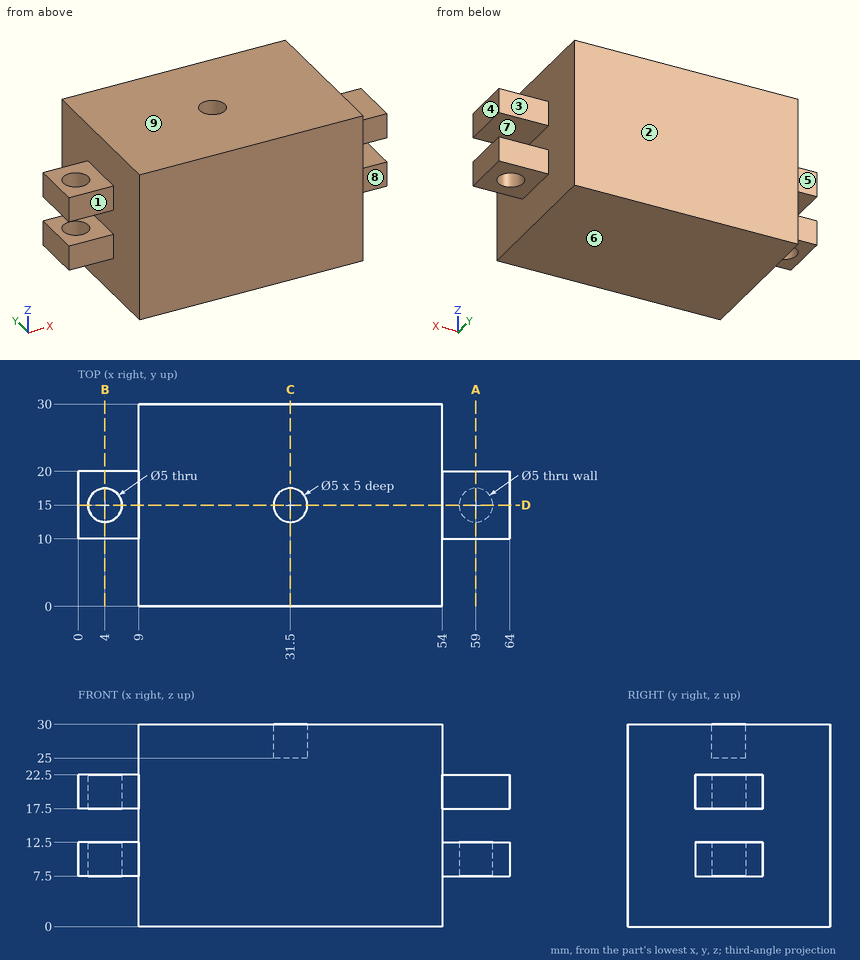
Print and shaded views of the part. All mm, measured from the part's lowest x, y and z. A direction names the side the tool comes from. Give positions to 0.01 mm unless a question says otherwise; leave off trailing zeros. Order: outer loops, then holes, each group sorted by start corner. A loop starts at its lowest first (then second) coordinate and runs counter-clockwise, first axis right, second up. Notation, with made-up numbers: (-28, 5) - (16, 5) arc R12 cw to (16, 28) - close; hole circle Ø4 at (78, 38.25). An arc over 180 degrees is marked (long way). Use a Markdown table: item, result.
1) 3-axis set-ups, long thin cutter, end or side, ignore diameter. For the marked faces 1, 2, 3, 4 and 5: which of +Z, -Z, +X, -X, +Y, -Y reach the whole face in a straight line?
Checked values:
| item | result |
|---|---|
| face 1 | +Z, -Z, -X, -Y |
| face 2 | +Z, -Z, +X, -X, +Y |
| face 3 | +Z, -Z, +X, +Y |
| face 4 | +Z, -Z, +X, +Y, -Y |
| face 5 | +Z, -Z, -X, +Y |
2) Flat gauge pins, fed straight in: P1, Ø4.5, axis at x = 4, y = 15, coming from the -Z side; P2, Ø2, axis at y = 25.5, z = 24.5, coming from the -X side; P3, Ø2.5, axis at x = 58.5, z = 9, coming from the +Y side; P4, Ø4, axis at y = 25.5, z = 20, coming from the +X side. Where does each tip first touch, or does it go through?
Checked values:
| item | result |
|---|---|
| P1 | through |
| P2 | x = 9 |
| P3 | y = 20 |
| P4 | x = 54 |
3) Saw through at B-B on x = 4. List the corners of the cut face in (y, z), plus the area to 3 significant figures.
Checked values:
| item | result |
|---|---|
| outline | (10, 7.5) - (12.5, 7.5) - (12.5, 12.5) - (10, 12.5) - close; (10, 17.5) - (12.5, 17.5) - (12.5, 22.5) - (10, 22.5) - close; (17.5, 7.5) - (20, 7.5) - (20, 12.5) - (17.5, 12.5) - close; (17.5, 17.5) - (20, 17.5) - (20, 22.5) - (17.5, 22.5) - close |
| area | 50.0 mm² |
4) Probe L1, parallel to X at y = 15, z = 10.4; L2, parallel to Y at x = 4, z = 21.2; L3, parallel to X at y = 15, z = 18.7. List the from-to ranges inside material, lowest first. Write a range as from..to.
Checked values:
| item | result |
|---|---|
| L1 | 0..1.5, 6.5..56.5, 61.5..64 |
| L2 | 10..12.5, 17.5..20 |
| L3 | 0..1.5, 6.5..64 |
5) Saw through at C-C on x = 31.5. List the corners of the cut face in (y, z).
Checked values:
| item | result |
|---|---|
| outline | (0, 0) - (30, 0) - (30, 30) - (17.5, 30) - (17.5, 25) - (12.5, 25) - (12.5, 30) - (0, 30) - close |
6) Saw through at D-D on y = 15. Count the separate pieces of the cut face and the enclosed holes in it, plus the area to 3 significant figures.
Checked values:
| item | result |
|---|---|
| separate pieces | 4 |
| enclosed holes | 0 |
| area | 1,440 mm² |
7) Two-plate mould, pull along Z, no slides. Class the marked faces 6, 7, 8 and 9: +Z half, -Z half, draft (parallel to the pull), parting line (faces both ways), or undercut.
Checked values:
| item | result |
|---|---|
| face 6 | -Z half |
| face 7 | undercut |
| face 8 | draft |
| face 9 | +Z half |
8) Saw through at A-A on x = 59. List the corners of the cut face in (y, z).
Checked values:
| item | result |
|---|---|
| outline | (10, 7.5) - (12.5, 7.5) - (12.5, 12.5) - (10, 12.5) - close; (10, 17.5) - (20, 17.5) - (20, 22.5) - (10, 22.5) - close; (17.5, 7.5) - (20, 7.5) - (20, 12.5) - (17.5, 12.5) - close |
